from build123d import *

# Parameters (mm, degrees)
SKETCH_1_W           = 40
SKETCH_1_H           = 40
EXTRUDE_1_DEPTH      = 20
EXTRUDE_2_DEPTH      = 7
EXTRUDE_2_DEPTH_BACK = 45
SKETCH_2_R           = 10
SKETCH_3_R           = 0.75
CUT_EXTRUDE_1_DEPTH  = 3


with BuildPart() as part:
    # 草图1 → 凸台-拉伸1 (new body)
    with BuildSketch(Plane(origin=(0, 0, 0), x_dir=(1, 0, 0), z_dir=(0, 1, 0))):
        with Locations((20, -20)):
            Rectangle(SKETCH_1_W, SKETCH_1_H)
    extrude(amount=EXTRUDE_1_DEPTH)

    # 草图2 → 凸台-拉伸2 (add, two sides: drawn at the far end of the back side and taken through both)
    with BuildSketch(Plane.XY.offset(40).offset(-EXTRUDE_2_DEPTH_BACK)):
        with Locations((10, 10)):
            Circle(SKETCH_2_R)
    extrude(amount=EXTRUDE_2_DEPTH + EXTRUDE_2_DEPTH_BACK)

    # 草图3 → 切除-拉伸1 (cut)
    with BuildSketch(Plane.XY.offset(40)):
        with Locations((31, 17)):
            Circle(SKETCH_3_R)
        with Locations((31, 3)):
            Circle(SKETCH_3_R)
    extrude(amount=-CUT_EXTRUDE_1_DEPTH, mode=Mode.SUBTRACT)


solid = part.part
Check sheet for the modelled part. Datum: model origin and axes. Units: mm. A direction names the side the tool comes from. Round coordinates to 2 decimals unless told otherwise and drop trailing zeros. Loops run counter-clockwise (first coordinate to the right, second up) from the corner with the lowest first, then second, coordinate; pieces in that order, holes last. Notation, with made-up numbers: M -4.5,66.5 L 1.5,66.5 A14 cw 1.5,87.5 Z; hole C 72,6.25 d8. An arc over 180 degrees is marked long. One line per item, written item: value.
(1) Release check for a two-part mould opening along X. For faces 4 (the face through (31, 17, 37)), 5 (the face through (31, 3, 37)), 6 (the face through (2, 2, 0)), 7 (the face through (40, 10, 20)) record: +X half, -X half, draft (parallel to the pull), parting line (faces both ways), or undercut.
Computed values:
face 4: undercut
face 5: undercut
face 6: draft
face 7: +X half
(2) Access from +Z, -Z, +X, -X, +Y, -Y to the whole of each face (thin tool, end or side, straight path). Record for faces 1 (the face through (31.69, 16.71, 38.52)), 2 (the face through (2, 2, 40)), 3 (the face through (2, 18, 40)).
Computed values:
face 1: +Z
face 2: +Z, -X, -Y
face 3: +Z, -X, +Y
(3) Sectioned sample at C-C, the plane x = 21. Record the cut outline in (y, z).
Computed values:
outline: M 0,0 L 20,0 L 20,40 L 0,40 Z
(4) Sectioned sample at A-A, the plane x = 16. Record the cut outline in (y, z), then the cut area to 3 significant figures.
Computed values:
outline: M 0,0 L 2,0 L 2,-5 L 18,-5 L 18,0 L 20,0 L 20,40 L 18,40 L 18,47 L 2,47 L 2,40 L 0,40 Z
area: 992 mm^2
(5) Sectioned sample at B-B, the plane y = 4.75. Record the cut outline in (x, z).
Computed values:
outline: M 0,0 L 1.49,0 L 1.49,-5 L 18.51,-5 L 18.51,0 L 40,0 L 40,40 L 18.51,40 L 18.51,47 L 1.49,47 L 1.49,40 L 0,40 Z
(6) Thickness scan on line 1 (Y direction, x = 31, z = 39); line 2 (Z direction, x = 20, y = 9). Record the ranges inside material, lowest first.
Computed values:
line 1: y = 0 to 2.25, 3.75 to 16.25, 17.75 to 20
line 2: z = 0 to 40
(7) Depth check by flat-ended pin: pin 1 Ø2 at (x, y) = (24, 15.5) entering from +Z; pin 2 Ø1.2 at (x, y) = (31, 3) entering from -Z; pin 3 Ø0.8 at (x, y) = (31, 3) entering from +Z. Enter the tip coordinate at first touch or a pass-through.
Computed values:
pin 1: stops at z = 40
pin 2: stops at z = 0
pin 3: stops at z = 37
